Verification items for the finished model (mm, model axes). Face numbers are marked on the shaded views. A direction names the side the tool comes from. Give positions to 0.01 mm unless a question says otherwise; leave off trailing zeros. Loops run counter-clockwise (first coordinate to the right, second up) from the corner with the lowest first, then second, coordinate; pieces in that order, holes last. Notation, with made-up numbers: (-12.5, -20.5) -> (17.5, -20.5) arc R25 ccw to (17.5, 0.5) -> close; hole circle Ø6 at (76.5, -29). An arc over 180 degrees is marked (long way). Answer in a Markdown table with one row per item. Add a question column.
Q1. Section check A-A on x = 5.25. Enter the section's corners in (y, z), and give its area (4 significant figures).
Q2. Section check D-D on z = -2.25. Enter the section's corners in (x, y), and give its area (3 significant figures).
Q3. Section check B-B on y = 3. Enter the section's corners in (x, z), and give its area (3 significant figures).
Q4. Material ranges on probe 1 along X at (y, z) = (5.5, 0.25); probe 2 along X at (y, z) = (10.25, -2); probe 3 along Z at (x, y) = (10, 6.95), recorded low to high.
Q5. Section check C-C on y = 8.25. Give the number of separate pieces and of enclosed holes in the cut face, and give its area (3 significant figures).
Q6. Set-up check for the marked faces 1, 2, 3, 4 and 5: record each of +Z, -Z, +X, -X, +Y, -Y from which the full face is reachable in a straight line by a thin tool's end or side.
Q7. Release check for a two-part mould opening along Z. For the marked faces 6, 7 and 8 record: pulls with the +Z half, pulls with the -Z half, needs draft (parallel to the pull), parting line crosses it, or undercut.
Q8. Gauge pin test, flat ends, axial feed: P1, Ø3, axis at x = 19.5, z = 0, coming from the -Y side; P2, Ø1.3, axis at x = 6, z = -3, coming from the +Y side; P3, Ø1.5, axis at y = 2.5, z = -2.5, coming from the +X side; P4, Ø0.8, axis at x = 10.5, z = -0.5, coming from the +Y side. Record the tip position at first contact, or that the pin passes through.
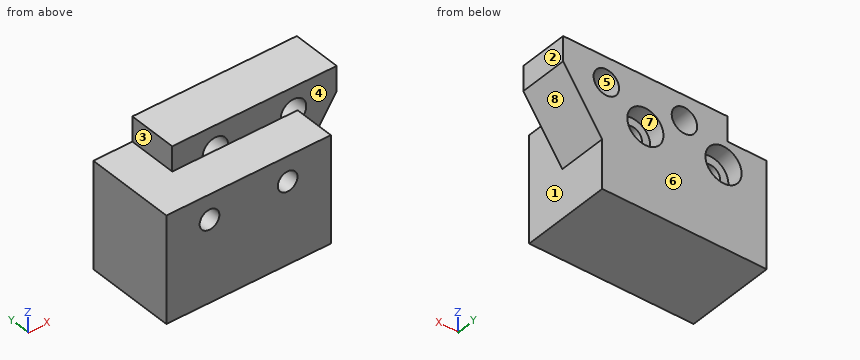
```python
from build123d import *

# Parameters (mm, degrees)
SKETCH1_W                      = 20
SKETCH1_H                      = 12.9
SKETCH1_R                      = 1.175
BOSS_EXTRUDE1_DEPTH            = 11
SKETCH2_W                      = 20
SKETCH2_H                      = 6
BOSS_EXTRUDE2_DEPTH            = 3
CBORE_FOR_M2_SHCS1_D           = 2.4
CBORE_FOR_M2_SHCS1_CBORE_D     = 4.4
CBORE_FOR_M2_SHCS1_CBORE_DEPTH = 2
CHAMFER1_SIZE2                 = 4.75
CHAMFER1_SIZE                  = 7
SKETCH5_R                      = 1.55
CUT_EXTRUDE1_DEPTH             = 6


with BuildPart() as part:
    # Sketch1 → Boss-Extrude1 (new body)
    with BuildSketch(Plane(origin=(0, 0, 0), x_dir=(1, 0, 0), z_dir=(0, 1, 0))):
        with Locations((10, 6.45)):
            Rectangle(SKETCH1_W, SKETCH1_H)
        with Locations(Location((5.25, 3, 0), (0, 0, 270))):
            Circle(SKETCH1_R, mode=Mode.SUBTRACT)
        with Locations(Location((14.75, 3, 0), (0, 0, 270))):
            Circle(SKETCH1_R, mode=Mode.SUBTRACT)
    extrude(amount=BOSS_EXTRUDE1_DEPTH)

    # Sketch2 → Boss-Extrude2 (add)
    with BuildSketch(Plane.XY):
        with Locations((14.75, 8)):
            Rectangle(SKETCH2_W, SKETCH2_H)
    extrude(amount=BOSS_EXTRUDE2_DEPTH)

    # CBORE for M2 SHCS1 (through all)
    with Locations(Plane(origin=(0, 11, 0), x_dir=(1, 0, 0), z_dir=(0, 1, 0))):
        with Locations((5.25, 3), (14.75, 3)):
            CounterBoreHole(CBORE_FOR_M2_SHCS1_D / 2, CBORE_FOR_M2_SHCS1_CBORE_D / 2, CBORE_FOR_M2_SHCS1_CBORE_DEPTH)

    # Chamfer1
    chamfer1_edges = [part.edges().sort_by_distance(p)[0] for p in [
        (20, 8, 0),
    ]]
    chamfer1_side = [part.faces().sort_by_distance(p)[0] for p in [
        (20, 8, -0.095),
    ]]
    chamfer(chamfer1_edges, length=CHAMFER1_SIZE - 0.0001, length2=CHAMFER1_SIZE2 - 0.0001, reference=chamfer1_side[0])  # a hair under: the kernel refuses the full size

    # Sketch5 → Cut-Extrude1 (cut)
    with BuildSketch(Plane(origin=(0, 11, 0), x_dir=(1, 0, 0), z_dir=(0, 1, 0))):
        with Locations(Location((10, 0, 0), (0, 0, 270))):
            Circle(SKETCH5_R)
        with Locations(Location((19.5, 0, 0), (0, 0, 270))):
            Circle(SKETCH5_R)
    extrude(amount=-CUT_EXTRUDE1_DEPTH, mode=Mode.SUBTRACT)


solid = part.part
```
Taken from the geometry:
| question | item | result |
|---|---|---|
| 1 | outline | (0, -12.9) -> (11, -12.9) -> (11, -5.2) -> (9, -5.2) -> (9, -4.2) -> (0, -4.2) -> close; (0, -1.8) -> (9, -1.8) -> (9, -0.8) -> (11, -0.8) -> (11, 3) -> (5, 3) -> (5, 0) -> (0, 0) -> close |
| 1 | area | 129.5 mm² |
| 2 | outline | (0, 0) -> (4.31, 0) -> (4.31, 9) -> (3.18, 9) -> (3.18, 11) -> (0, 11) -> close; (6.19, 0) -> (13.81, 0) -> (13.81, 9) -> (12.68, 9) -> (12.68, 11) -> (7.32, 11) -> (7.32, 9) -> (6.19, 9) -> close; (15.69, 0) -> (20, 0) -> (20, 5) -> (23.22, 5) -> (23.22, 11) -> (16.82, 11) -> (16.82, 9) -> (15.69, 9) -> close |
| 2 | area | 189 mm² |
| 3 | outline | (0, -12.9) -> (20, -12.9) -> (20, 0) -> (0, 0) -> close; hole circle Ø2.4 at (5.25, -3); hole circle Ø2.4 at (14.75, -3) |
| 3 | area | 249 mm² |
| 4 | probe 1 | x = 4.75 to 8.47, 11.53 to 17.97, 21.03 to 24.75 |
| 4 | probe 2 | x = 0 to 3.29, 7.21 to 12.79, 16.71 to 23.39 |
| 4 | probe 3 | z = -12.9 to -1.55, 1.55 to 3 |
| 5 | separate pieces | 1 |
| 5 | enclosed holes | 4 |
| 5 | area | 310 mm² |
| 6 | face 1 | -Z, +X, -Y |
| 6 | face 2 | +Z, -Z, +X, +Y, -Y |
| 6 | face 3 | +Z, -X, +Y, -Y |
| 6 | face 4 | +Z, +X, -Y |
| 6 | face 5 | +Y |
| 7 | face 6 | needs draft |
| 7 | face 7 | undercut |
| 7 | face 8 | pulls with the -Z half |
| 8 | P1 | stops at y = 0 |
| 8 | P2 | stops at y = 9 |
| 8 | P3 | stops at x = 20 |
| 8 | P4 | stops at y = 5 |
